Input: part model. Units: mm. Frame: model coordinates. Face numbers are marked on the shaded views. Give positions to 0.01 mm unless a question says otherwise; leave off trailing zeros. Order: outer loops, then holes, each group sorted by start corner. A loop starts at its lowest first (then second) coordinate and runs counter-clockwise, first axis right, second up.
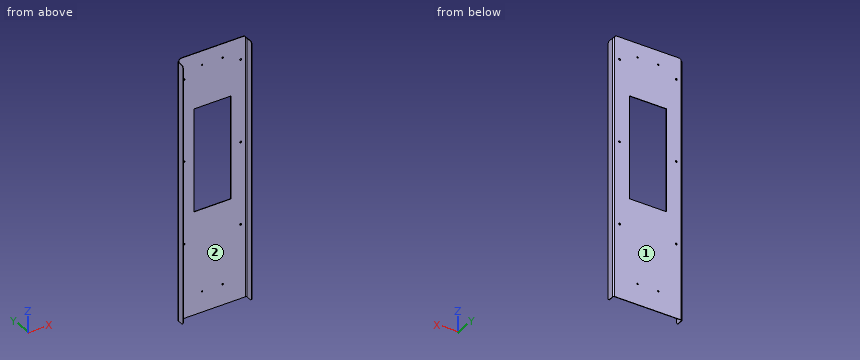
```python
from build123d import *

# Parameters (mm, degrees)
SKETCH_1_W                  = 323
SKETCH_1_H                  = 1268
SKETCH_1_R                  = 4.5
SKETCH_1_R_2                = 3.5
SKETCH_1_W_2                = 180
SKETCH_1_H_2                = 500
SM_BASE_FLANGE_1_DEPTH      = 2
SM_EDGE_FLANGE_1_DEPTH      = 1256
SM_EDGE_FLANGE_1_BEND_DEPTH = 1256
FILLET_1_R                  = 10
FILLET_2_R                  = 10


# Sheet-metal steps are written as plain solids
with BuildPart() as part:
    # Sketch 1 → Базовая кромка1 (new body)
    with BuildSketch(Plane(origin=(0, 0, 0), x_dir=(1, 0, 0), z_dir=(0, 1, 0))):
        Rectangle(SKETCH_1_W, SKETCH_1_H)
        with Locations(Location((-137.5, -526, 0), (0, 0, 270))):
            Circle(SKETCH_1_R, mode=Mode.SUBTRACT)
        with Locations(Location((137.5, -526, 0), (0, 0, 270))):
            Circle(SKETCH_1_R, mode=Mode.SUBTRACT)
        with Locations(Location((-137.5, -126, 0), (0, 0, 270))):
            Circle(SKETCH_1_R, mode=Mode.SUBTRACT)
        with Locations(Location((137.5, -126, 0), (0, 0, 270))):
            Circle(SKETCH_1_R, mode=Mode.SUBTRACT)
        with Locations(Location((-137.5, 274, 0), (0, 0, 270))):
            Circle(SKETCH_1_R, mode=Mode.SUBTRACT)
        with Locations(Location((137.5, 274, 0), (0, 0, 270))):
            Circle(SKETCH_1_R, mode=Mode.SUBTRACT)
        with Locations(Location((-50, -566, 0), (0, 0, 270))):
            Circle(SKETCH_1_R_2, mode=Mode.SUBTRACT)
        with Locations(Location((50, -566, 0), (0, 0, 270))):
            Circle(SKETCH_1_R_2, mode=Mode.SUBTRACT)
        with Locations(Location((-50, 534, 0), (0, 0, 270))):
            Circle(SKETCH_1_R_2, mode=Mode.SUBTRACT)
        with Locations(Location((50, 534, 0), (0, 0, 270))):
            Circle(SKETCH_1_R_2, mode=Mode.SUBTRACT)
        with Locations((0, -116)):
            Rectangle(SKETCH_1_W_2, SKETCH_1_H_2, mode=Mode.SUBTRACT)
    extrude(amount=-SM_BASE_FLANGE_1_DEPTH)

    # Ребро-кромка1 section (across the edge) → Ребро-кромка1 (add)
    with BuildSketch(Plane(origin=(165.5, -2, -634), x_dir=(-1, 0, 0), z_dir=(0, 0, 1))):
        with BuildLine():
            Line((-2, 4), (-2, 38))
            Line((-2, 38), (0, 38))
            Line((0, 38), (0, 4))
            ThreePointArc((0, 4), (1.171572875, 1.171572875), (4, 0))
            Line((4, 0), (4, -2))
            ThreePointArc((4, -2), (-0.242640687, -0.242640687), (-2, 4))
        make_face()
    extrude(amount=SM_EDGE_FLANGE_1_DEPTH)

    # Ребро-кромка1 section 2 (across the edge) → Ребро-кромка1 bend (add)
    with BuildSketch(Plane(origin=(-165.5, -2, 622), x_dir=(1, 0, 0), z_dir=(0, 0, -1))):
        with BuildLine():
            Line((-2, 4), (-2, 38))
            Line((-2, 38), (0, 38))
            Line((0, 38), (0, 4))
            ThreePointArc((0, 4), (1.171572875, 1.171572875), (4, 0))
            Line((4, 0), (4, -2))
            ThreePointArc((4, -2), (-0.242640687, -0.242640687), (-2, 4))
        make_face()
    extrude(amount=SM_EDGE_FLANGE_1_BEND_DEPTH)

    # Скругление1
    fillet_1_edges = [part.edges().sort_by_distance(p)[0] for p in [
        (-166.5, -40, 622),
        (-166.5, -40, -634),
        (166.5, -40, -634),
        (166.5, -40, 622),
    ]]
    fillet(fillet_1_edges, radius=FILLET_1_R)

    # Скругление2
    fillet_2_edges = [part.edges().sort_by_distance(p)[0] for p in [
        (161.5, -1, 634),
        (-161.5, -1, 634),
    ]]
    fillet(fillet_2_edges, radius=FILLET_2_R)


solid = part.part
```
1) First-contact query: P1, Ø6, axis at x = -112, z = -322, coming from the +Y side; P2, Ø1, axis at y = -0.5, z = 49.5, coming from the +X side; P3, Ø6.5, axis at x = -163.5, y = -16, coming from the +Z side; P4, Ø1.6, axis at y = -1, z = 622.5, coming from the -X side. Flat tips, straight axial feed; report the tip coordinate or a pass-through.
2) Cut plane A-A (x = 77). Return the cut outline in (y, z), then the cut area to 3 significant figures.
3) Line query: probe 1 along X at (y, z) = (-14, 394); probe 2 along X at (y, z) = (-0.6, 126); probe 3 along X at (y, z) = (-1.3, -534). Output: solid intervals per line, ascending.
4) Cut plane C-C (y = -16.5). Return the cut outline in (x, z).
5) Cut plane B-B (z = 66). Return the cut outline in (x, y), then the cut area to 3 significant figures.
6) Cut plane D-D (z = -433). Return the cut outline in (x, y), then the cut area to 3 significant figures.
7) Pull-direction query (X, two-part tool) for the marked faces 1 and 2; classes: pulls with the +X half, pulls with the -X half, needs draft (parallel to the pull), parting line crosses it, or undercut.
Geometry says:
1. P1: stops at y = 0
1. P2: stops at x = 164.82
1. P3: stops at z = 622
1. P4: stops at x = -165.61
2. outline: (-2, -634) - (0, -634) - (0, -134) - (-2, -134) - close; (-2, 366) - (0, 366) - (0, 634) - (-2, 634) - close
2. area: 1,540 mm2
3. probe 1: x = -167.5 to -165.5, 165.5 to 167.5
3. probe 2: x = -164.12 to -142, -133 to -90, 90 to 133, 142 to 164.12
3. probe 3: x = -165.23 to -53.5, -46.5 to 46.5, 53.5 to 165.23
4. outline: (-167.5, -634) - (-165.5, -634) - (-165.5, 622) - (-167.5, 622) - close; (165.5, -634) - (167.5, -634) - (167.5, 622) - (165.5, 622) - close
5. outline: (-167.5, -40) - (-165.5, -40) - (-165.5, -6) arc R4 cw to (-161.5, -2) - (-90, -2) - (-90, 0) - (-161.5, 0) arc R6 ccw to (-167.5, -6) - close; (90, -2) - (161.5, -2) arc R4 cw to (165.5, -6) - (165.5, -40) - (167.5, -40) - (167.5, -6) arc R6 ccw to (161.5, 0) - (90, 0) - close
5. area: 453 mm2
6. outline: (-167.5, -40) - (-165.5, -40) - (-165.5, -6) arc R4 cw to (-161.5, -2) - (161.5, -2) arc R4 cw to (165.5, -6) - (165.5, -40) - (167.5, -40) - (167.5, -6) arc R6 ccw to (161.5, 0) - (-161.5, 0) arc R6 ccw to (-167.5, -6) - close
6. area: 813 mm2
7. face 1: needs draft
7. face 2: undercut
